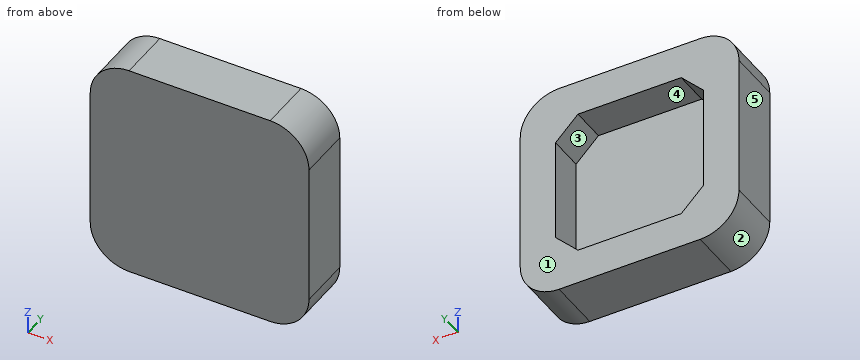
```python
from build123d import *

# Parameters (mm, degrees)
SKETCH1_W           = 62
SKETCH1_H           = 62
SKETCH1_W_2         = 42
SKETCH1_H_2         = 42
BOSS_EXTRUDE1_DEPTH = 10
SKETCH2_W           = 62
SKETCH2_H           = 62
BOSS_EXTRUDE2_DEPTH = 5
FILLET1_R           = 11


with BuildPart() as part:
    # Sketch1 → Boss-Extrude1 (new body)
    # profile 1 of 5: a face of its own
    with BuildSketch(Plane(origin=(0, 0, 0), x_dir=(1, 0, 0), z_dir=(0, 1, 0))):
        Rectangle(SKETCH1_W, SKETCH1_H)
        Rectangle(SKETCH1_W_2, SKETCH1_H_2, mode=Mode.SUBTRACT)
    # profile 2 of 5: a face of its own
    with BuildSketch(Plane(origin=(0, 0, 0), x_dir=(1, 0, 0), z_dir=(0, 1, 0))):
        Polygon((21, -21), (21, -14.636038969), (14.636038969, -21), align=None)
    # profile 3 of 5: a face of its own
    with BuildSketch(Plane(origin=(0, 0, 0), x_dir=(1, 0, 0), z_dir=(0, 1, 0))):
        Polygon((14.636038969, 21), (21, 14.636038969), (21, 21), align=None)
    # profile 4 of 5: a face of its own
    with BuildSketch(Plane(origin=(0, 0, 0), x_dir=(1, 0, 0), z_dir=(0, 1, 0))):
        Polygon((-21, 14.636038969), (-14.636038969, 21), (-21, 21), align=None)
    # profile 5 of 5: a face of its own
    with BuildSketch(Plane(origin=(0, 0, 0), x_dir=(1, 0, 0), z_dir=(0, 1, 0))):
        Polygon((-21, -21), (-14.636038969, -21), (-21, -14.636038969), align=None)
    extrude(amount=BOSS_EXTRUDE1_DEPTH)

    # Sketch2 → Boss-Extrude2 (add)
    with BuildSketch(Plane(origin=(0, 0, 0), x_dir=(-1, 0, 0), z_dir=(0, -1, 0))):
        Rectangle(SKETCH2_W, SKETCH2_H)
    extrude(amount=BOSS_EXTRUDE2_DEPTH)

    # Fillet1
    fillet1_edges = [part.edges().sort_by_distance(p)[0] for p in [
        (-31, 2.5, 31),
        (-31, 2.5, -31),
        (31, 2.5, -31),
        (31, 2.5, 31),
    ]]
    fillet(fillet1_edges, radius=FILLET1_R)


solid = part.part
```
Input: part model. Units: mm. Frame: model coordinates. Face numbers are marked on the shaded views. A direction names the side the tool comes from. Round coordinates to 2 decimals unless told otherwise and drop trailing zeros. Loops run counter-clockwise (first coordinate to the right, second up) from the corner with the lowest first, then second, coordinate; pieces in that order, holes last.
1) Set-up query: the marked faces 4 and 5. Return all of +Z, -Z, +X, -X, +Y, -Y with unobstructed straight access to the full face (end or side cutting, diameter ignored); none if empty.
Ans:
face 4: +Y
face 5: +Z, -Z, -X, +Y, -Y
2) Material intervals for line 1 (Z direction, x = -11, y = 3); line 2 (Y direction, x = -12, z = -11.5), sorted ascending.
Ans:
line 1: z = -31 to -21, 21 to 31
line 2: y = -5 to 0
3) Section query D-D on x = -24.5. Return the cut outline in (y, z), plus the area to 3 significant figures.
Ans:
outline: (-5, -30.04) - (10, -30.04) - (10, 30.04) - (-5, 30.04) - close
area: 901 mm2
4) Section query C-C on z = -1.5. Return the cut outline in (x, y).
Ans:
outline: (-31, -5) - (31, -5) - (31, 10) - (21, 10) - (21, 0) - (-21, 0) - (-21, 10) - (-31, 10) - close
5) Section query B-B on x = -0.5. Return the cut outline in (y, z).
Ans:
outline: (-5, -31) - (10, -31) - (10, -21) - (0, -21) - (0, 21) - (10, 21) - (10, 31) - (-5, 31) - close
6) Pin query (flat end, axial travel): pin 1 (12.5 mm diameter, centred on x = 3.5, z = 3.5, fed in from +Y). Return the tip coordinate at first contact, or that it passes through.
Ans:
pin 1: stops at y = 0
7) Pull-direction query (Z, two-part tool) for the marked faces 1, 2 and 3; classes: released by +Z, released by -Z, zero draft, split by the parting line, or undercut.
Ans:
face 1: zero draft
face 2: released by -Z
face 3: undercut
8) Section query A-A on y = 7.75. Return the cut outline in (x, z).
Ans:
outline: (-31, -20) arc R11 ccw to (-20, -31) - (20, -31) arc R11 ccw to (31, -20) - (31, 20) arc R11 ccw to (20, 31) - (-20, 31) arc R11 ccw to (-31, 20) - close; hole (-21, -14.64) - (-14.64, -21) - (14.64, -21) - (21, -14.64) - (21, 14.64) - (14.64, 21) - (-14.64, 21) - (-21, 14.64) - close
